Autodesk Inventor part; units mm, degrees
ref_plane "YZ Plane" through (0, 0, 0) normal (1, 0, 0) x (0, 1, 0)
ref_plane "XZ Plane" through (0, 0, 0) normal (0, 1, 0) x (-1, 0, 0)
ref_plane "XY Plane" through (0, 0, 0) normal (0, 0, 1) x (1, 0, 0)
sketch "Sketch1" plane through (0, 0, 0) normal (0, 0, 1) x (1, 0, 0)
  line L0 (-3.9016, 5.1111) -> (32.0984, 5.1111)
  line L1 (35.0984, 2.1111) -> (35.0984, -33.8889)
  line L2 (32.0984, -36.8889) -> (-3.9016, -36.8889)
  line L3 (-6.9016, -33.8889) -> (-6.9016, 2.1111)
  circle A0 centre (14.0984, -15.8889) radius 11
  line L4 (35.0984, 2.1111) -> (32.0984, 5.1111)
  line L5 (-6.9016, 2.1111) -> (-3.9016, 5.1111)
  line L6 (-6.9016, -33.8889) -> (-3.9016, -36.8889)
  line L7 (35.0984, -33.8889) -> (32.0984, -36.8889)
  circle A1 centre (30.8484, -32.6389) radius 1.25
  circle A2 centre (-2.6516, -32.6389) radius 1.25
  circle A3 centre (-2.6516, 0.8611) radius 1.25
  circle A4 centre (30.8484, 0.8611) radius 1.25
  point P0 (0, 0)
extrude "Extrusion8" add sketch "Sketch1" along normal blind 5
sketch "Sketch2" plane through (35.0984, -33.8889, 0) normal (1, 0, 0) x (0, 0, -1)
  circle A0 centre (-2.5, 26) radius 1.5
  point P0 (0, 33.8889)
  point P1 (-5, -3)
hole "Hole1" at (35.0984, -7.8889, 2.5) direction (-1, 0, 0) diameter 3 depth 5 tip angle 118
sketch "Sketch3" plane through (-6.9016, -33.8889, 0) normal (-1, 0, 0) x (0, 0, 1)
  circle A0 centre (2.5, 26) radius 1.5
  circle A1 centre (2.5, 26) radius 1.5
  point P0 (0, 33.8889)
hole "Hole3" at (-6.9016, -7.8889, 2.5) direction (1, 0, 0) diameter 3 depth 5 tip angle 118
thread "Thread1"
thread "Thread2"
properties part number "attachment motor" material "Lead"
Read the model definition and answer for the solid it produces. Units are mm, in the model's axes. Coordinates: 2 decimals unless noted, no trailing zeros. Order: outer loops, then holes, each group sorted by start corner. A loop starts at its lowest first (then second) coordinate and runs counter-clockwise, first axis right, second up. Notation, with made-up numbers: M 89.5,47 L 107.5,47 A9 cw 107.5,56 Z; hole C -29,29 d7. An arc over 180 degrees is marked long. Put each result on its own line as item: value. Start each with the question number.
Item 1: Section B-B, the plane x = 21 is taken. Determine the outline of the cut face in (y, z).
Item 2: The mould has two halves that part along Z. Classify faces 1 (the face through (4, -25, 0)), 2 (the face through (32.563, -9.376, 2.695)), 3 (the face through (-5.42, -35.37, 2.46)), 4 (the face through (29.354, -7.811, 2.252)): +Z half, -Z half, draft (parallel to the pull), parting line (faces both ways), or undercut.
Item 3: Section A-A, the plane y = -23 is taken. Determine the outline of the cut face in (x, z), plus the area to 3 significant figures.
Item 4: Section C-C, the plane z = 3.5 is taken. Count the separate pieces of the cut face and the enclosed holes in it, plus the area to 3 significant figures.
Item 5: Consider probe 1 along X at (y, z) = (0, 0.95); probe 2 along X at (y, z) = (-10.5, 1.7); probe 3 along X at (y, z) = (-20, 3.95). Determine where each line is inside the solid, lowest interval first. Write a range as [from, to].
Computed:
1. outline: M -36.89,0 L -24.45,0 L -24.45,5 L -36.89,5 Z; M -7.32,0 L 5.11,0 L 5.11,5 L -7.32,5 Z
2. face 1: -Z half
2. face 2: undercut
2. face 3: draft
2. face 4: undercut
3. outline: M -6.9,0 L 5.71,0 L 5.71,5 L -6.9,5 Z; M 22.49,0 L 35.1,0 L 35.1,5 L 22.49,5 Z
3. area: 126 mm2
4. separate pieces: 1
4. enclosed holes: 5
4. area: 1,320 mm2
5. probe 1: x = [-6.9, -3.56], [-1.75, 29.94], [31.75, 35.1]
5. probe 2: x = [-6.9, 4.51], [23.69, 35.1]
5. probe 3: x = [-6.9, 3.9], [24.3, 35.1]
